Geometry: final body of the model. Coordinates: model frame, mm. A direction names the side the tool comes from. Coordinates: 2 decimals unless noted, no trailing zeros. Order: outer loops, then holes, each group sorted by start corner. A loop starts at its lowest first (then second) coordinate and runs counter-clockwise, first axis right, second up. Notation, with made-up numbers: (67, 67) -> (123, 67) arc R29 cw to (123, 92) -> close; hole circle Ø7 at (56, -18.5). An arc over 180 degrees is marked (long way). Answer in a Markdown table with one row per item. Add a question column.
1) Ray query, line 1 (X direction, y = -21.25, z = 101.6); line 2 (Z direction, x = 0, y = -14); line 3 (Z direction, x = 0, y = -22). Return the intervals inside material, ascending. Write a range as from..to.
2) Pull-direction query (Z, two-part tool) for faces 1 (the face through (1, -39, 0)), 2 (the face through (12.4, -19.05, 97.6)), 3 (the face through (12.7, -70, 16)); classes: +Z half, -Z half, draft (parallel to the pull), parting line (faces both ways), or undercut.
3) Section query C-C on z = 11. Return the cut outline in (x, y), then the cut area to 3 significant figures.
4) Section query B-B on y = -68.5. Return the cut outline in (x, z).
5) Set-up query: faces 4 (the face through (1, -39, 25.4)), 5 (the face through (-2.48, -22.269, 120.488)), 6 (the face through (-50.8, -33, 47)), 7 (the face through (19.05, -70, 29)), 8 (the face through (38.1, -33, 47)). Return all of +Z, -Z, +X, -X, +Y, -Y with unobstructed straight access to the full face (end or side cutting, diameter ignored); none if empty.
6) Section query A-A on x = 0. Return the cut outline in (y, z), then the cut area to 3 significant figures.
7) Section query D-D on x = -21. Return the cut outline in (y, z), then the cut area to 3 significant figures.
8) Contact query for flat-ended pins moving along their axis: P1, Ø1.5, axis at x = 53, z = 88, coming from the -Y side; P2, Ø12.5, axis at y = -36, z = 45.5, coming from the +X side; P3, Ø1.5, axis at y = -67, z = 28.5, coming from the -X side; P4, Ø16, axis at x = 0.5, y = -59, coming from the +Z side. Output: stop coordinate, or through.
```python
from build123d import *

# Parameters (mm, degrees)
F1_DEPTH = 76.2
F3_DEPTH = 25.401
F4_R     = 12.7
F5_DEPTH = 25.401
F4_R_2   = 19.05
F6_DEPTH = 6.35
F9_DEPTH = 6.35
F11_W    = 6.35
F11_H    = 6.35


with BuildPart() as f1:
    # F0 (on Right) → F1 (new body, symmetric)
    with BuildSketch(Plane.YZ):
        Polygon((-76.2, 0), (0, 0), (0, 152.4), (-25.4, 152.4), (-25.4, 25.4), (-76.2, 25.4), align=None)
    extrude(amount=F1_DEPTH, both=True)

    # F2 (on face) → F3 (cut, through all)
    with BuildSketch(Plane.XY.offset(25.4)):
        with BuildLine():
            Line((12.7, -76.2), (12.7, -63.5))
            ThreePointArc((12.7, -63.5), (0, -50.8), (-12.7, -63.5))
            Line((-12.7, -63.5), (-12.7, -76.2))
            Line((-12.7, -76.2), (12.7, -76.2))
        make_face()
    extrude(amount=-F3_DEPTH, mode=Mode.SUBTRACT)

    # F4 (on face) → F5 (cut, through all)
    with BuildSketch(Plane.XZ.offset(25.4)):
        with Locations((0, 101.6)):
            Circle(F4_R)
    extrude(amount=-F5_DEPTH, mode=Mode.SUBTRACT)

    # F4 (on face) → F6 (cut)
    with BuildSketch(Plane.XZ.offset(25.4)):
        with Locations((0, 101.6)):
            Circle(F4_R_2)
        with Locations((0, 101.6)):
            Circle(F4_R, mode=Mode.SUBTRACT)
    extrude(amount=-F6_DEPTH, mode=Mode.SUBTRACT)

    # F8 (on offset) → F9 (join, symmetric)
    with BuildSketch(Plane.YZ.offset(44.45)):
        Polygon((-50.8, 25.4), (-25.4, 25.4), (-25.4, 101.6), align=None)
    extrude(amount=F9_DEPTH, both=True)

    # F10: F1 across plane


with BuildPart() as f1_1:
    add(f1.part)
    add(f1.part.mirror(Plane.YZ))

    # F12: sweep along a path in F2
    with BuildLine(Plane.XY.offset(25.4)) as f12_path:
        Line((-12.7, -76.2), (-12.7, -63.5))
        ThreePointArc((-12.7, -63.5), (0, -50.8), (12.7, -63.5))
        Line((12.7, -63.5), (12.7, -76.2))
    # F11 (on face) → F12 (sweep)
    with BuildSketch(Plane.XZ.offset(76.2)):
        with Locations((-15.875, 28.575)):
            Rectangle(F11_W, F11_H)
    sweep(path=f12_path.line)


solid = f1_1.part
```
Result:
| question | item | result |
|---|---|---|
| 1 | line 1 | -76.2..-19.05, 19.05..76.2 |
| 1 | line 2 | 0..88.9, 114.3..152.4 |
| 1 | line 3 | 0..82.55, 120.65..152.4 |
| 2 | face 1 | -Z half |
| 2 | face 2 | undercut |
| 2 | face 3 | draft |
| 3 | outline | (-76.2, -76.2) -> (-12.7, -76.2) -> (-12.7, -63.5) arc R12.7 cw to (12.7, -63.5) -> (12.7, -76.2) -> (76.2, -76.2) -> (76.2, 0) -> (-76.2, 0) -> close |
| 3 | area | 11,000 mm2 |
| 4 | outline | (-76.2, 0) -> (-12.7, 0) -> (-12.7, 31.75) -> (-19.05, 31.75) -> (-19.05, 25.4) -> (-76.2, 25.4) -> close; (12.7, 0) -> (76.2, 0) -> (76.2, 25.4) -> (19.05, 25.4) -> (19.05, 31.75) -> (12.7, 31.75) -> close |
| 5 | face 4 | +Z |
| 5 | face 5 | -Y |
| 5 | face 6 | +Z, -X, -Y |
| 5 | face 7 | +Z, +X, -Y |
| 5 | face 8 | +Z, -Y |
| 6 | outline | (-50.8, 0) -> (0, 0) -> (0, 88.9) -> (-19.05, 88.9) -> (-19.05, 82.55) -> (-25.4, 82.55) -> (-25.4, 25.4) -> (-44.45, 25.4) -> (-44.45, 31.75) -> (-50.8, 31.75) -> close; (-25.4, 120.65) -> (-19.05, 120.65) -> (-19.05, 114.3) -> (0, 114.3) -> (0, 152.4) -> (-25.4, 152.4) -> close |
| 6 | area | 3,830 mm2 |
| 7 | outline | (-76.2, 0) -> (0, 0) -> (0, 152.4) -> (-25.4, 152.4) -> (-25.4, 25.4) -> (-76.2, 25.4) -> close |
| 7 | area | 5,160 mm2 |
| 8 | P1 | y = -25.4 |
| 8 | P2 | x = 50.8 |
| 8 | P3 | x = -19.05 |
| 8 | P4 | through |
